Job drawing, mm, ordinate dimensions from the low corner. One solid piece. Give positions to 0.01 mm unless a question says otherwise; leave off trailing zeros. Loops run counter-clockwise (first coordinate to the right, second up) from the corner with the lowest first, then second, coordinate; pieces in that order, holes last. Notation, with made-up numbers: (-1.75, 81.25) - (4.25, 81.25) arc R23 cw to (4.25, 112.25) - close; hole circle Ø3 at (27, 17). An arc over 180 degrees is marked (long way). Answer as CSV lines item,"result". Start each with the question number.
Item 1: Drill centre line: L1, parallel to X at y = 5, z = 23.5. Where is it in solid material? Low to high. Write a range as from..to.
Item 2: Saw through at A-A on x = 8. Give the cut face in (y, z), plus the area to 3 significant figures.
Item 3: Pin check, flat tips, straight feed: pin 1 (8 mm diameter, centred on y = 24.5, z = 14, fed in from +X); pin 2 (2.5 mm diameter, centred on x = 8.5, y = 46.5, fed in from +Z). Stop position of each tip, or through.
Item 4: Saw through at B-B on y = 12.5. Give the cut face in (x, z), plus the area to 3 significant figures.
Item 5: Saw through at C-C on z = 31.5. Give the cut face in (x, y), plus the area to 3 significant figures.
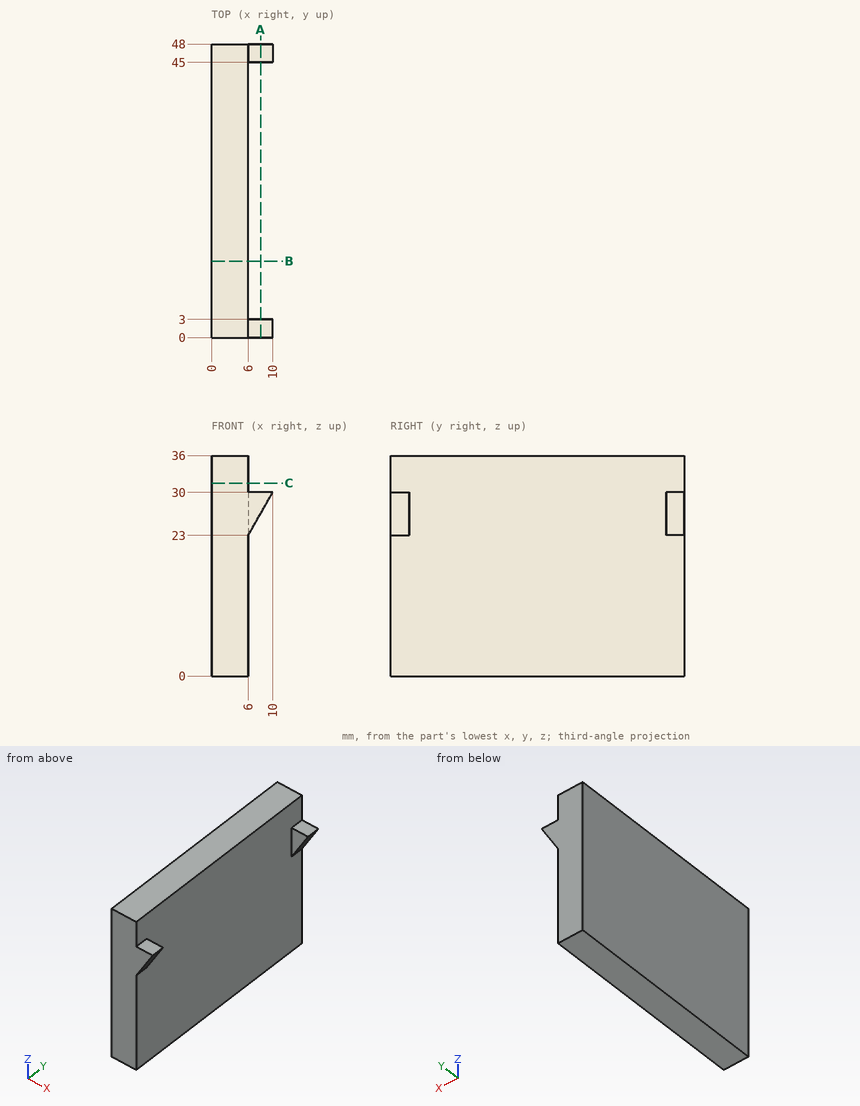
Responses:
1,L1,"0..6"
2,outline,"(0, 26.5) - (3, 26.5) - (3, 30) - (0, 30) - close; (45, 26.5) - (48, 26.5) - (48, 30) - (45, 30) - close"
2,area,"21.0 mm2"
3,pin 1,"x = 6"
3,pin 2,"z = 30"
4,outline,"(0, 0) - (6, 0) - (6, 36) - (0, 36) - close"
4,area,"216 mm2"
5,outline,"(0, 0) - (6, 0) - (6, 48) - (0, 48) - close"
5,area,"288 mm2"
